from build123d import *

# Parameters (mm, degrees)
SKETCH1_W           = 25.4
SKETCH1_H           = 25.4
BOSS_EXTRUDE1_DEPTH = 254
FILLET1_R           = 1.5875
HOLE1_OUTLINE_R     = 2.5527
HOLE1_DEPTH         = 254
SKETCH7_W           = 6.5278
SKETCH7_H           = 2.2352
CUT_EXTRUDE2_DEPTH  = 254
FILLET4_R           = 0.396875
CIRPATTERN2_DEPTH   = 254


# Read off the part's stored shape, not the designer's step: Hole1, CirPattern2
with BuildPart() as part:
    # Sketch1 → Boss-Extrude1 (new body)
    with BuildSketch(Plane.XY):
        Rectangle(SKETCH1_W, SKETCH1_H)
    extrude(amount=BOSS_EXTRUDE1_DEPTH)

    # Fillet1
    fillet1_edges = [part.edges().sort_by_distance(p)[0] for p in [
        (12.7, -12.7, 127),
        (-12.7, -12.7, 127),
        (-12.7, 12.7, 127),
        (12.7, 12.7, 127),
    ]]
    fillet(fillet1_edges, radius=FILLET1_R)

    # Hole1 outline → Hole1 (cut)
    with BuildSketch(Plane.XY):
        with Locations((0, -0.048792482)):
            Circle(HOLE1_OUTLINE_R)
    extrude(amount=HOLE1_DEPTH, mode=Mode.SUBTRACT)

    # Sketch7 → Cut-Extrude2 (cut)
    with BuildSketch(Plane.XY.offset(254)):
        with Locations((0, 11.5824)):
            Rectangle(SKETCH7_W, SKETCH7_H)
        Polygon((-3.175, 4.5212), (-7.3025, 10.4648), (7.3025, 10.4648), (3.175, 4.5212), align=None)
    extrude(amount=-CUT_EXTRUDE2_DEPTH, mode=Mode.SUBTRACT)

    # Fillet4
    fillet4_edges = [part.edges().sort_by_distance(p)[0] for p in [
        (-3.2639, 10.4648, 127),
        (-3.2639, 12.7, 127),
        (3.2639, 12.7, 127),
        (3.2639, 10.4648, 127),
    ]]
    fillet(fillet4_edges, radius=FILLET4_R)

    # CirPattern2 outline → CirPattern2 (cut)
    with BuildSketch(Plane.XY):
        with BuildLine():
            ThreePointArc((-3.660775, -10.562384964), (-3.380141996, -10.67862696), (-3.2639, -10.959259964))
            Line((-3.2639, -10.959259964), (-3.2639, -12.7))
            Line((-3.2639, -12.7), (3.2639, -12.7))
            Line((3.2639, -12.7), (3.2639, -10.959259964))
            ThreePointArc((3.2639, -10.959259964), (3.380141996, -10.67862696), (3.660775, -10.562384964))
            Line((3.660775, -10.562384964), (7.3025, -10.562384964))
            Line((7.3025, -10.562384964), (3.175, -4.618784964))
            Line((3.175, -4.618784964), (-3.175, -4.618784964))
            Line((-3.175, -4.618784964), (-7.3025, -10.562384964))
            Line((-7.3025, -10.562384964), (-3.660775, -10.562384964))
        make_face()
        with BuildLine():
            Line((-12.7, -3.312692482), (-10.910467482, -3.312692482))
            ThreePointArc((-10.910467482, -3.312692482), (-10.629834478, -3.428934478), (-10.513592482, -3.709567482))
            Line((-10.513592482, -3.709567482), (-10.513592482, -7.351292482))
            Line((-10.513592482, -7.351292482), (-4.569992482, -3.223792482))
            Line((-4.569992482, -3.223792482), (-4.569992482, 3.126207518))
            Line((-4.569992482, 3.126207518), (-10.513592482, 7.253707518))
            Line((-10.513592482, 7.253707518), (-10.513592482, 3.611982518))
            ThreePointArc((-10.513592482, 3.611982518), (-10.629834478, 3.331349514), (-10.910467482, 3.215107518))
            Line((-10.910467482, 3.215107518), (-12.7, 3.215107518))
            Line((-12.7, 3.215107518), (-12.7, -3.312692482))
        make_face()
        with BuildLine():
            ThreePointArc((10.513592482, -3.709567482), (10.629834478, -3.428934478), (10.910467482, -3.312692482))
            Line((10.910467482, -3.312692482), (12.7, -3.312692482))
            Line((12.7, -3.312692482), (12.7, 3.215107518))
            Line((12.7, 3.215107518), (10.910467482, 3.215107518))
            ThreePointArc((10.910467482, 3.215107518), (10.629834478, 3.331349514), (10.513592482, 3.611982518))
            Line((10.513592482, 3.611982518), (10.513592482, 7.253707518))
            Line((10.513592482, 7.253707518), (4.569992482, 3.126207518))
            Line((4.569992482, 3.126207518), (4.569992482, -3.223792482))
            Line((4.569992482, -3.223792482), (10.513592482, -7.351292482))
            Line((10.513592482, -7.351292482), (10.513592482, -3.709567482))
        make_face()
    extrude(amount=CIRPATTERN2_DEPTH, mode=Mode.SUBTRACT)


solid = part.part
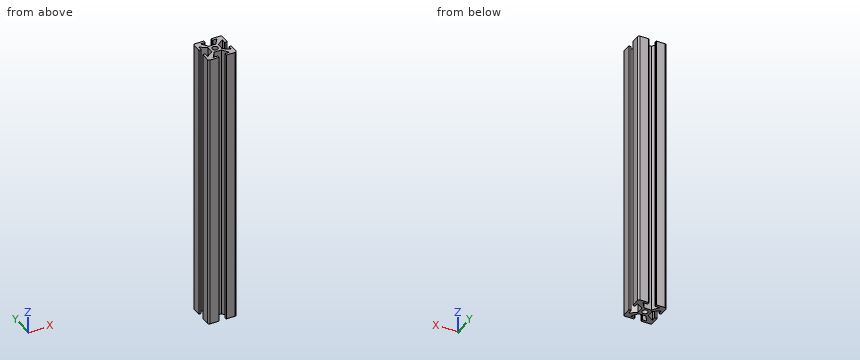
Part model, mm, in its own coordinate system. Give positions to 0.01 mm unless a question says otherwise; leave off trailing zeros. Write each loop counter-clockwise with the first axis right and the second up, starting at its lowest first coordinate (ties: lowest second). Pieces come first, ordered by that corner, then holes.
1) Probe L1, parallel to X at y = -4.25, z = 224.5; L2, parallel to X at y = -0.5, z = 140.5; L3, parallel to Y at x = 0, z = 51. List the from-to ranges inside material, lowest first.
Resolved:
L1: x = -12.7 to -10.51, -6.05 to 6.05, 10.51 to 12.7
L2: x = -4.57 to -2.51, 2.51 to 4.57
L3: y = -4.62 to -2.6, 2.5 to 4.52
2) Cut at A-A on x = 0. Write the cut outline in (y, z), then the cut area to 3 significant figures.
Resolved:
outline: (-4.62, 0) - (-2.6, 0) - (-2.6, 254) - (-4.62, 254) - close; (2.5, 0) - (4.52, 0) - (4.52, 254) - (2.5, 254) - close
area: 1,020 mm2
3) Pin check, flat tips, straight feed: pin 1 (0.5 mm diameter, centred on x = 12, z = 177.5, fed in from -Y); pin 2 (3 mm diameter, centred on x = -0.5, z = 90, fed in from +Y); pin 3 (1 mm diameter, centred on x = -4.5, y = -9.5, fed in from -Z). Stop position of each tip, or through.
Resolved:
pin 1: stops at y = -12.57
pin 2: stops at y = 4.52
pin 3: passes through
